Build history of the part. All positions in model axes, mm. Round coordinates to 2 decimals unless told otherwise and drop trailing zeros. Write each loop counter-clockwise with the first axis right and the second up, starting at its lowest first coordinate (ties: lowest second). Pieces come first, ordered by that corner, then holes. Notation, with made-up numbers: (3.5, 76) - (44.5, 76) arc R10 cw to (44.5, 91) - close; hole circle Ø9 at (2, -23). An arc over 180 degrees is marked (long way). Answer as a JSON object with one key per item and string values. Group by question number.
Item 1: Slice it at A-A, the plane x = 0. List the corners of the cut face in (y, z), then the cut area to 3 significant figures.
Item 2: Probe line 1 (Y direction, x = 0, z = 1.2); line 2 (X direction, y = -10, z = 1.2); line 3 (Y direction, x = -12, z = 1.45). List the from-to ranges inside material, lowest first. Write a range as from..to.
Item 3: Flat gauge pins, fed straight in: pin 1 (1 mm diameter, centred on y = 9, z = 2, fed in from -X); pin 2 (4 mm diameter, centred on x = 8.5, y = -2, fed in from +Z); pin 3 (1 mm diameter, centred on x = 2.5, z = 1.5, fed in from -Y). Where does each tip first touch, or does it go through?
Item 4: Two-plate mould, pull along Y, no slides. Class faces 1 (the cylindrical face through (-3.27, -14.74, 1.49)), 2 (the cylindrical face through (-1.269, 9.667, 0.197)), 3 (the flat face through (3, -10, 0)): +Y half, -Y half, draft (parallel to the pull), parting line (faces both ways), or undercut.
Item 5: Slice it at C-C, the plane z = 0.9. List the corners of the cut face in (x, y).
from build123d import *

# Parameters (mm, degrees)
F0_R     = 15.1
F0_R_2   = 9.75
F1_DEPTH = 2.5
F2_R     = 14.65
F3_DEPTH = 2.1
F4_R     = 0.5


with BuildPart() as f1:
    # F0 (on Top) → F1 (new body)
    with BuildSketch(Plane.XY):
        Circle(F0_R)
        Circle(F0_R_2, mode=Mode.SUBTRACT)
    extrude(amount=F1_DEPTH)

    # F2 (on face) → F3 (cut)
    with BuildSketch(Plane.XY.offset(2.5)):
        Circle(F2_R)
    extrude(amount=-F3_DEPTH, mode=Mode.SUBTRACT)

    # F4
    f4_edges = [f1.edges().sort_by_distance(p)[0] for p in [
        (-15.1, 0, 0),
    ]]
    fillet(f4_edges, radius=F4_R)


solid = f1.part
Geometry says:
{
 "1": {"outline": "(-15.1, 0.5) arc R0.5 ccw to (-14.6, 0) - (-9.75, 0) - (-9.75, 0.4) - (-14.65, 0.4) - (-14.65, 2.5) - (-15.1, 2.5) - close; (9.75, 0) - (14.6, 0) arc R0.5 ccw to (15.1, 0.5) - (15.1, 2.5) - (14.65, 2.5) - (14.65, 0.4) - (9.75, 0.4) - close", "area": "6.06 mm^2"},
 "2": {"line 1": "y = -15.1..-14.65, 14.65..15.1", "line 2": "x = -11.31..-10.71, 10.71..11.31", "line 3": "y = -9.17..-8.4, 8.4..9.17"},
 "3": {"pin 1": "stops at x = -12.48", "pin 2": "stops at z = 0.4", "pin 3": "stops at y = -14.97"},
 "4": {"face 1": "parting line", "face 2": "undercut", "face 3": "draft"},
 "5": {"outline": "circle Ø30.2 at (0, 0); hole circle Ø29.3 at (0, 0)"}
}
